```python
from build123d import *

# Parameters (mm, degrees)
F0_W      = 304.8
F0_H      = 304.8
F1_DEPTH  = 50.8
F2_R      = 25.4
F3_DEPTH  = 304.8
F6_W      = 38.1
F6_H      = 304.8
F7_DEPTH  = 609.6
F8_R      = 25.4
F9_R      = 25.4
F10_R     = 25.4
F11_R     = 68.2122039911
F12_DEPTH = 38.1
F13_R     = 63.8417796902
F14_DEPTH = 38.1
F15_W     = 76.0798454285
F15_H     = 198.4691917896
F16_DEPTH = 38.1
F17_R     = 12.7


with BuildPart() as f1:
    # F0 (on Front) → F1 (new body)
    with BuildSketch(Plane.XZ):
        Rectangle(F0_W, F0_H)
    extrude(amount=F1_DEPTH)

    # F2 (on face) → F3 (join)
    with BuildSketch(Plane.XZ.offset(50.8)):
        with Locations((-101.6, 101.6)):
            Circle(F2_R)
    extrude(amount=F3_DEPTH)


with BuildPart() as f4_1:
    # F4: instance of F1
    add(f1.part.mirror(Plane.XY))


with BuildPart() as f1_1:
    add(f1.part)

    add(f4_1.part)  # F5 merges F4_1
    # F5: F1, F4_1 across plane
    add(f1.part.mirror(Plane.YZ))
    add(f4_1.part.mirror(Plane.YZ))

    # F6 (on face) → F7 (join)
    with BuildSketch(Plane(origin=(0, 0, 0), x_dir=(-1, 0, 0), z_dir=(0, 1, 0))):
        with Locations((133.35, 0)):
            Rectangle(F6_W, F6_H)
    extrude(amount=F7_DEPTH)

    # F8
    f8_edges = [f1_1.edges().sort_by_distance(p)[0] for p in [
        (-133.35, 609.6, 152.4),
        (-133.35, 609.6, -152.4),
    ]]
    fillet(f8_edges, radius=F8_R)

    # F9
    f9_edges = [f1_1.edges().sort_by_distance(p)[0] for p in [
        (-114.3, 0, 0),
        (152.4, -25.4, 152.4),
    ]]
    fillet(f9_edges, radius=F9_R)

    # F10
    f10_edges = [f1_1.edges().sort_by_distance(p)[0] for p in [
        (152.4, -25.4, -152.4),
    ]]
    fillet(f10_edges, radius=F10_R)

    # F11 (on face) → F12 (cut, through all)
    with BuildSketch(Plane.YZ.offset(-114.3)):
        with Locations((175.7188588381, 0)):
            Circle(F11_R)
    extrude(amount=-F12_DEPTH, mode=Mode.SUBTRACT)

    # F13 (on face) → F14 (cut, through all)
    with BuildSketch(Plane.YZ.offset(-114.3)):
        with Locations((363.809466362, 0)):
            Circle(F13_R)
    extrude(amount=-F14_DEPTH, mode=Mode.SUBTRACT)

    # F15 (on face) → F16 (cut, through all)
    with BuildSketch(Plane.YZ.offset(-114.3)):
        with Locations((519.2769765854, 0)):
            Rectangle(F15_W, F15_H)
    extrude(amount=-F16_DEPTH, mode=Mode.SUBTRACT)

    # F17
    f17_edges = [f1_1.edges().sort_by_distance(p)[0] for p in [
        (-133.35, 557.316899, -99.234596),
        (-133.35, 557.316899, 99.234596),
        (-133.35, 481.237054, 99.234596),
        (-133.35, 481.237054, -99.234596),
    ]]
    fillet(f17_edges, radius=F17_R)


solid = f1_1.part
```
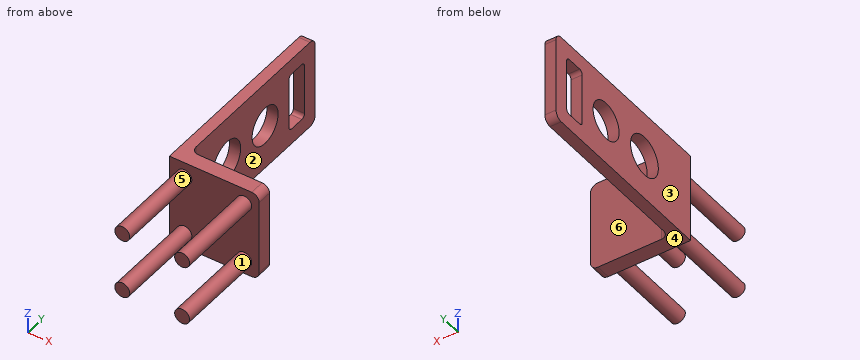
Verification items for the finished model (mm, model axes). Face numbers are marked on the shaded views. A direction names the side the tool comes from. Coordinates: 2 decimals unless noted, no trailing zeros. Order: outer loops, then holes, each group sorted by start corner. A loop starts at its lowest first (then second) coordinate and runs counter-clockwise, first axis right, second up. Notation, with made-up numbers: (-24, 42) -> (-12, 42) arc R15 cw to (-12, 61) -> close; hole circle Ø6 at (41.5, 32.5). An arc over 180 degrees is marked (long way). Answer as CSV lines item,"result". Start each with the question number.
1) Cross-section at B-B, the plane z = -48. Record the boundary of the cut face in (x, y), then the cut area to 3 significant figures.
2) Gauge pin test, flat ends, axial feed: pin 1 Ø1 at (y, z) = (182.5, 71.5) entering from +X; pin 2 Ø1 at (x, z) = (100.5, 53) entering from +Y; pin 3 Ø11.5 at (x, z) = (-127.5, 41) entering from -Y. Record the tip position at first contact, or that the pin passes through.
3) Material ranges on L1, parallel to Y at x = 101, z = -45; L2, parallel to X at y = 433.5, z = 129; L3, parallel to X at y = -207.5, z = -105, recorded low to high. Write a range as [from, to].
4) Release check for a two-part mould opening along Z. For the marked faces 4, 5 and 6 record: released by +Z, released by -Z, zero draft, split by the parting line, or undercut.
5) Set-up check for the marked faces 1, 2 and 3: record each of +Z, -Z, +X, -X, +Y, -Y from which the full face is reachable in a straight line by a thin tool's end or side.
6) Cross-section at A-A, the plane y = 514. Record the boundary of the cut face in (x, z), then the cut area to 3 significant figures.
7) Cross-section at C-C, the plane x = 101.6. Record the boundary of the cut face in (y, z).
8) Cross-section at D-D, the plane y = 365.5. Record the boundary of the cut face in (x, z), then the cut area to 3 significant figures.
Conclusion:
1,outline,"(-152.4, -50.8) -> (152.4, -50.8) -> (152.4, 0) -> (-88.9, 0) arc R25.4 cw to (-114.3, 25.4) -> (-114.3, 127.25) -> (-152.4, 127.25) -> close; (-152.4, 224.18) -> (-114.3, 224.18) -> (-114.3, 321.72) -> (-152.4, 321.72) -> close; (-152.4, 405.9) -> (-114.3, 405.9) -> (-114.3, 481.24) -> (-152.4, 481.24) -> close; (-152.4, 557.32) -> (-114.3, 557.32) -> (-114.3, 609.6) -> (-152.4, 609.6) -> close"
1,area,"29,000 mm²"
2,pin 1,"stops at x = -114.3"
2,pin 2,"stops at y = 0"
2,pin 3,"stops at y = -50.8"
3,L1,"y = [-50.8, 0]"
3,L2,"x = [-152.4, -114.3]"
3,L3,"x = [-126.77, -76.43], [76.43, 126.77]"
4,face 4,"released by -Z"
4,face 5,"undercut"
4,face 6,"zero draft"
5,face 1,"-Y"
5,face 2,"+Z, -Z, +X, +Y"
5,face 3,"+Z, -Z, -X, +Y, -Y"
6,outline,"(-152.4, -152.4) -> (-114.3, -152.4) -> (-114.3, -99.23) -> (-152.4, -99.23) -> close; (-152.4, 99.23) -> (-114.3, 99.23) -> (-114.3, 152.4) -> (-152.4, 152.4) -> close"
6,area,"4,050 mm²"
7,outline,"(-355.6, -127) -> (-50.8, -127) -> (-50.8, -152.4) -> (0, -152.4) -> (0, 152.4) -> (-50.8, 152.4) -> (-50.8, 127) -> (-355.6, 127) -> (-355.6, 76.2) -> (-50.8, 76.2) -> (-50.8, -76.2) -> (-355.6, -76.2) -> close"
8,outline,"(-152.4, -152.4) -> (-114.3, -152.4) -> (-114.3, -63.82) -> (-152.4, -63.82) -> close; (-152.4, 63.82) -> (-114.3, 63.82) -> (-114.3, 152.4) -> (-152.4, 152.4) -> close"
8,area,"6,750 mm²"
